Here's how the part is built. I have some questions about the finished solid (model axes, mm). A direction names the side the tool comes from. Give positions to 0.01 mm unless a question says otherwise; leave off trailing zeros. Loops run counter-clockwise (first coordinate to the right, second up) from the corner with the lowest first, then second, coordinate; pieces in that order, holes last.
Q1. Suppose I cut it at A-A (y = 1.2). List the corners of the cut face in (x, z) for me.
Q2. I'm going to push flat-ended pins straight in: P1, Ø1.2, axis at y = 3, z = -16.5, coming from the +X side; P2, Ø7.5, axis at x = 0, z = 0, coming from the +Y side; P3, Ø5.5, axis at x = 3.8, z = -15.5, coming from the +Y side; P4, Ø6.5, axis at x = 25, z = 0, coming from the -Y side. Where does each tip first touch, or does it pass through?
Q3. Suppose I cut it at D-D (x = -8.5). List the corners of the cut face in (y, z) for me, and give its area (3 significant figures).
Q4. I need wall thicknesses on probe 1 along Z at (x, y) = (0, 2.45); probe 2 along Z at (x, y) = (0, 2.2); probe 3 along Z at (x, y) = (-14, 2.85). Which ranges of each line are inside material? Lowest first, please.
Q5. For faces 5 (the face through (-12, 2, 16)), 6 (the face through (-13, 2, -17)), 7 (the face through (16, 2, -15)), 8 (the face through (3, 2.262, 0)), 9 (the face through (12, 2, 16)), which set-ups out of +Z, -Z, +X, -X, +Y, -Y let a thin tool reach every point of the face, with its end or its side?
Q6. Suppose I cut it at C-C (x = 1). List the corners of the cut face in (y, z) for me, and give its area (3 significant figures).
Q7. Thinking about a two-plate mould opening in X: for faces 1 (the face through (-0.54, 1.15, 2.44)), 2 (the face through (0, 2, 20)), 3 (the face through (3.575, 2.348, -13.787)), 4 (the face through (-25, 2.4, -9.9)), which applies, pulls with the +X half, pulls with the -X half, needs draft (parallel to the pull), parting line crosses it, or undercut?
Q8. Suppose I cut it at B-B (x = 25). List the corners of the cut face in (y, z) for me, and give its area (3 significant figures).
```python
from build123d import *

# Parameters (mm, degrees)
SKETCH1_W             = 65
SKETCH1_H             = 45
BOSS_EXTRUDE1_DEPTH   = 4.7625
SKETCH2_R             = 2.5
CUT_EXTRUDE1_DEPTH    = 5.7625
F_8_32_TAPPED_HOLE1_D = 3.4544
SKETCH6_R             = 3.96875
CUT_EXTRUDE2_DEPTH    = 5.7625
CUT_EXTRUDE3_DEPTH    = 5.7625
SKETCH9_R             = 6.35
CUT_EXTRUDE4_DEPTH    = 2.5


with BuildPart() as part:
    # Sketch1 → Boss-Extrude1 (new body)
    with BuildSketch(Plane(origin=(0, 0, 0), x_dir=(1, 0, 0), z_dir=(0, 1, 0))):
        Rectangle(SKETCH1_W, SKETCH1_H)
    extrude(amount=BOSS_EXTRUDE1_DEPTH)

    # Sketch2 → Cut-Extrude1 (cut, through all)
    with BuildSketch(Plane(origin=(0, 4.7625, 0), x_dir=(1, 0, 0), z_dir=(0, 1, 0))):
        Circle(SKETCH2_R)
    extrude(amount=-CUT_EXTRUDE1_DEPTH, mode=Mode.SUBTRACT)

    # #8-32 Tapped Hole1 (through all)
    with Locations(Plane(origin=(-15.76090252, 4.7625, 28.427239646), x_dir=(-1, 0, 0), z_dir=(0, 1, 0))):
        with Locations((-31.26090252, -24.627239646), (-1.76090252, -28.427239646), (-19.56090252, -43.927239646), (-15.76090252, -12.427239646)):
            Hole(F_8_32_TAPPED_HOLE1_D / 2)

    # Sketch6 → Cut-Extrude2 (cut, through all)
    with BuildSketch(Plane(origin=(0, 4.7625, 0), x_dir=(1, 0, 0), z_dir=(0, 1, 0))):
        with Locations((-25, 0)):
            Circle(SKETCH6_R)
        with Locations((25, 0)):
            Circle(SKETCH6_R)
    extrude(amount=-CUT_EXTRUDE2_DEPTH, mode=Mode.SUBTRACT)

    # Sketch8 → Cut-Extrude3 (cut, through all)
    with BuildSketch(Plane(origin=(0, 4.7625, 0), x_dir=(1, 0, 0), z_dir=(0, 1, 0))):
        with BuildLine():
            Line((6, -16), (18.899494937, -16))
            Line((18.899494937, -16), (29.949747468, -4.949747468))
            ThreePointArc((29.949747468, -4.949747468), (32, 0), (29.949747468, 4.949747468))
            Line((29.949747468, 4.949747468), (19.899494937, 15))
            Line((19.899494937, 15), (13, 15))
            Line((13, 15), (13, 19))
            Line((13, 19), (0, 19))
            Line((0, 19), (0, 22.5))
            Line((0, 22.5), (32.5, 22.5))
            Line((32.5, 22.5), (32.5, -22.5))
            Line((32.5, -22.5), (0, -22.5))
            Line((0, -22.5), (0, -20))
            Line((0, -20), (4.472135955, -20))
            ThreePointArc((4.472135955, -20), (5.605034154, -18.140932539), (6, -16))
        make_face()
    cut_extrude3 = extrude(amount=-CUT_EXTRUDE3_DEPTH, mode=Mode.SUBTRACT)

    # Mirror1: Cut-Extrude3 across plane
    add(cut_extrude3.mirror(Plane(origin=(0, 0, 0), x_dir=(0, 0, 1), z_dir=(1, 0, 0))), mode=Mode.SUBTRACT)

    # Sketch9 → Cut-Extrude4 (cut)
    with BuildSketch(Plane(origin=(0, 4.7625, 0), x_dir=(1, 0, 0), z_dir=(0, 1, 0))):
        Circle(SKETCH9_R)
    extrude(amount=-CUT_EXTRUDE4_DEPTH, mode=Mode.SUBTRACT)


solid = part.part
```
Solutions:
1. outline: (-29.95, -4.95) - (-19.9, -15) - (-13, -15) - (-13, -19) - (13, -19) - (13, -15) - (19.9, -15) - (29.95, -4.95) arc R7 ccw to (29.95, 4.95) - (18.9, 16) - (6, 16) arc R6 ccw to (4.47, 20) - (-4.47, 20) arc R6 ccw to (-6, 16) - (-18.9, 16) - (-29.95, 4.95) arc R7 ccw to start; hole circle Ø7.94 at (-25, 0); hole circle Ø3.45 at (-14, 0); hole circle Ø5 at (0, 0); hole circle Ø3.45 at (0, 16); hole circle Ø3.45 at (3.8, -15.5); hole circle Ø3.45 at (15.5, 3.8); hole circle Ø7.94 at (25, 0)
2. P1: stops at x = 13
2. P2: stops at y = 2.26
2. P3: stops at y = 4.76
2. P4: passes through
3. outline: (0, -19) - (4.76, -19) - (4.76, 16) - (0, 16) - close
3. area: 167 mm2
4. probe 1: z = -19 to -6.35, 6.35 to 14.27, 17.73 to 20
4. probe 2: z = -19 to -2.5, 2.5 to 14.27, 17.73 to 20
4. probe 3: z = -15 to -1.73, 1.73 to 16
5. face 5: +Z, -X, +Y, -Y
5. face 6: -Z, -X, +Y, -Y
5. face 7: -Z, +X, +Y, -Y
5. face 8: +Y
5. face 9: +Z, +X, +Y, -Y
6. outline: (0, -19) - (4.76, -19) - (4.76, -6.27) - (2.26, -6.27) - (2.26, -2.29) - (0, -2.29) - close; (0, 2.29) - (2.26, 2.29) - (2.26, 6.27) - (4.76, 6.27) - (4.76, 14.59) - (0, 14.59) - close; (0, 17.41) - (4.76, 17.41) - (4.76, 20) - (0, 20) - close
6. area: 131 mm2
7. face 1: undercut
7. face 2: needs draft
7. face 3: undercut
7. face 4: pulls with the -X half
8. outline: (0, -9.9) - (4.76, -9.9) - (4.76, -3.97) - (0, -3.97) - close; (0, 3.97) - (4.76, 3.97) - (4.76, 9.9) - (0, 9.9) - close
8. area: 56.5 mm2
